Part model, mm, in its own coordinate system. A direction names the side the tool comes from. Round coordinates to 2 decimals unless told otherwise and drop trailing zeros. Write each loop counter-clockwise with the first axis right and the second up, starting at its lowest first coordinate (ties: lowest second). Pieces come first, ordered by that corner, then holes. Notation, with made-up numbers: M -17,67.5 L 2,67.5 A22 cw 2,75.5 Z; hole C 72.25,34 d10. An arc over 180 degrees is marked long. Use a Markdown table: item, result. Add a question column.
1) Which spindle directions (+Z, -Z, +X, -X, +Y, -Y) get a long thin tool onto all of the face, cutting with end or side? Do faces 1 (the face through (-144.436, 3.131, 146.069)), 2 (the face through (-137.062, 3.131, 135.482)). Say none if no direction does.
2) Wall check: probe 1 along X at (y, z) = (1, 64.5); probe 2 along X at (y, z) = (3.75, 178); probe 3 along Z at (x, y) = (34, 0.5). Give the ranges that are in metal, low to high.
3) Drop flat-ended pins along their axis: P1, Ø1.5, axis at x = 38, y = 3.5, coming from the -Z side; P2, Ø2, axis at x = 99.5, y = 5.5, coming from the -Z side; P3, Ø2, axis at x = 95.5, y = 1, coming from the -Z side. Give the stop position or say it passes through.
4) Slice it at D-D on x = -12. Write the cut outline in (y, z).
5) Slice it at C-C on z = 176.5. Write the cut outline in (x, y).
6) Slice it at B-B on y = 2.75. Write the cut outline in (x, z), plus the area to 3 significant figures.
7) Slice it at A-A on z = -101. Write the cut outline in (x, y).
```python
from build123d import *

# Parameters (mm, degrees)
BOSS_EXTRUDE1_DEPTH = 6.35


with BuildPart() as part:
    # Sketch1 → Boss-Extrude1 (new body)
    with BuildSketch(Plane(origin=(0, 0, 0), x_dir=(1, 0, 0), z_dir=(0, 1, 0))):
        with BuildLine():
            Line((-192.717689271, 135.886792847), (-192.717689271, -79.826280605))
            Line((-192.717689271, -79.826280605), (-79.826280605, -192.717689271))
            Line((-79.826280605, -192.717689271), (79.826280605, -192.717689271))
            Line((79.826280605, -192.717689271), (192.717689271, -79.826280605))
            Line((192.717689271, -79.826280605), (192.717689271, 135.886792847))
            Line((192.717689271, 135.886792847), (199.067689271, 135.886792847))
            ThreePointArc((199.067689271, 135.886792847), (203.557817332, 134.026920908), (205.417689271, 129.536792847))
            Line((205.417689271, 129.536792847), (205.417689271, 85.086792847))
            Line((205.417689271, 85.086792847), (205.417689271, -82.456536726))
            ThreePointArc((205.417689271, -82.456536726), (204.934324303, -84.886576522), (203.557817332, -86.946664787))
            Line((203.557817332, -86.946664787), (86.946664787, -203.557817332))
            ThreePointArc((86.946664787, -203.557817332), (84.886576522, -204.934324303), (82.456536726, -205.417689271))
            Line((82.456536726, -205.417689271), (-82.456536726, -205.417689271))
            ThreePointArc((-82.456536726, -205.417689271), (-84.886576522, -204.934324303), (-86.946664787, -203.557817332))
            Line((-86.946664787, -203.557817332), (-203.557817332, -86.946664787))
            ThreePointArc((-203.557817332, -86.946664787), (-204.934324303, -84.886576522), (-205.417689271, -82.456536726))
            Line((-205.417689271, -82.456536726), (-205.417689271, 85.086792847))
            Line((-205.417689271, 85.086792847), (-205.417689271, 129.536792847))
            ThreePointArc((-205.417689271, 129.536792847), (-203.557817332, 134.026920908), (-199.067689271, 135.886792847))
            Line((-199.067689271, 135.886792847), (-192.717689271, 135.886792847))
        make_face()
    extrude(amount=BOSS_EXTRUDE1_DEPTH)


solid = part.part
```
Entries:
| question | item | result |
|---|---|---|
| 1 | face 1 | +Z, -X, +Y, -Y |
| 1 | face 2 | -Z, +Y, -Y |
| 2 | probe 1 | x = -205.42 to -192.72, 192.72 to 205.42 |
| 2 | probe 2 | x = -112.5 to -94.54, 94.54 to 112.5 |
| 2 | probe 3 | z = 192.72 to 205.42 |
| 3 | P1 | stops at z = 192.72 |
| 3 | P2 | stops at z = 172.04 |
| 3 | P3 | stops at z = 176.04 |
| 4 | outline | M 0,192.72 L 6.35,192.72 L 6.35,205.42 L 0,205.42 Z |
| 5 | outline | M -114,0 L -96.04,0 L -96.04,6.35 L -114,6.35 Z; M 96.04,0 L 114,0 L 114,6.35 L 96.04,6.35 Z |
| 6 | outline | M -205.42,-129.54 A6.35 ccw -199.07,-135.89 L -192.72,-135.89 L -192.72,79.83 L -79.83,192.72 L 79.83,192.72 L 192.72,79.83 L 192.72,-135.89 L 199.07,-135.89 A6.35 ccw 205.42,-129.54 L 205.42,82.46 A6.35 ccw 203.56,86.95 L 86.95,203.56 A6.35 ccw 82.46,205.42 L -82.46,205.42 A6.35 ccw -86.95,203.56 L -203.56,86.95 A6.35 ccw -205.42,82.46 Z |
| 6 | area | 11,800 mm^2 |
| 7 | outline | M -205.42,0 L -192.72,0 L -192.72,6.35 L -205.42,6.35 Z; M 192.72,0 L 205.42,0 L 205.42,6.35 L 192.72,6.35 Z |
